from build123d import *

# Parameters (mm, degrees)
CIRPATTERN1_COUNT = 3


with BuildPart() as part:
    # Sketch1 → Revolve1 (revolve)
    with BuildSketch(Plane.XY):
        with BuildLine():
            Line((-9.525, 6.494310079), (-9.525, 0))
            Line((-9.525, 0), (0, 0))
            Line((0, 0), (0, 11.02868))
            Line((0, 11.02868), (-2.615161836, 11.02868))
            ThreePointArc((-2.615161836, 11.02868), (-3.1664948, 10.980444616), (-3.701075791, 10.837204071))
            Line((-3.701075791, 10.837204071), (-7.435913955, 9.47783415))
            ThreePointArc((-7.435913955, 9.47783415), (-8.950807741, 8.315415264), (-9.525, 6.494310079))
        make_face()
    revolve(axis=Axis((0, -0.551434, 0), (0, 1, 0)))

    # Sketch2 → #4-40 Tapped Hole1 (revolve, cut)
    with BuildSketch(Plane(origin=(0, 0, 5.715), x_dir=(0, 0, -1), z_dir=(1, 0, 0))):
        Polygon((0, 0), (0, 9.188152758), (1.1303, 8.509), (1.1303, 0), align=None)
    f_4_40_tapped_hole1 = revolve(axis=Axis((0, -6.35, 5.715), (0, 1, 0)), mode=Mode.SUBTRACT)

    # CirPattern1: #4-40 Tapped Hole1 ×3 about axis
    cirpattern1_axis = Axis((0, 0, 0), (0, 1, 0))
    for i in range(1, CIRPATTERN1_COUNT):
        add(f_4_40_tapped_hole1.rotate(cirpattern1_axis, i * 360 / CIRPATTERN1_COUNT), mode=Mode.SUBTRACT)


solid = part.part
Part model, mm, in its own coordinate system. A direction names the side the tool comes from. Give positions to 0.01 mm unless a question says otherwise; leave off trailing zeros. Write each loop counter-clockwise with the first axis right and the second up, starting at its lowest first coordinate (ties: lowest second). Pieces come first, ordered by that corner, then holes.
1) Cut at B-B on y = 9.75. Write the cut outline in (x, z), then the cut area to 3 significant figures.
Resolved:
outline: circle Ø13.38 at (0, 0)
area: 141 mm2
2) Cut at C-C on y = 8. Write the cut outline in (x, z) (1 decimal).
Resolved:
outline: circle Ø18.3 at (0, 0); hole circle Ø2.3 at (-4.9, -2.9); hole circle Ø2.3 at (0, 5.7); hole circle Ø2.3 at (4.9, -2.9)
3) Probe L1, parallel to X at y = 8, z = -2.5; L2, parallel to X at y = 2.5, z = -2.25; L3, parallel to Z at x = -5.75, y = 4. List the from-to ranges inside material, lowest first.
Resolved:
L1: x = -8.8 to -6.02, -3.88 to 3.88, 6.02 to 8.8
L2: x = -9.26 to -5.9, -4 to 4, 5.9 to 9.26
L3: z = -7.59 to -3.66, -2.06 to 7.59
4) Which spindle directions (+Z, -Z, +X, -X, +Y, -Y) get a long thin tool onto all of the face, cutting with end or side? Do faces 4 (the face through (-4.26, 4.19, -1.96)), 5 (the face through (0, 0, 0)). Say none if no direction does.
Resolved:
face 4: -Y
face 5: +Z, -Z, +X, -X, -Y
5) Two-plate mould, pull along Z, no slides. Class faces 1 (the face through (0.853, 10.752, -3.841)), 2 (the face through (-5.144, 9.07, -2.832)), 3 (the face through (0, 11.029, 0)): released by +Z, released by -Z, zero draft, split by the parting line, or undercut.
Resolved:
face 1: split by the parting line
face 2: undercut
face 3: zero draft
6) Cut at A-A on y = 1.25. State how many separate pieces and enclosed holes the cut face has, then the cut area to 3 significant figures.
Resolved:
separate pieces: 1
enclosed holes: 3
area: 273 mm2
7) Pin check, flat tips, straight feed: pin 1 (1.8 mm diameter, centred on x = -4.95, z = -2.86, fed in from -Y); pin 2 (4 mm diameter, centred on y = 5, z = 4, fed in from +X); pin 3 (1 mm diameter, centred on y = 5, z = -6.5, fed in from -X). Stop position of each tip, or through.
Resolved:
pin 1: stops at y = 8.65
pin 2: stops at x = 9.31
pin 3: stops at x = -7.4
